Model file for the job. Use its own axes, mm. A direction names the side the tool comes from. Round coordinates to 2 decimals unless told otherwise and drop trailing zeros. Loops run counter-clockwise (first coordinate to the right, second up) from the corner with the lowest first, then second, coordinate; pieces in that order, holes last. Notation, with made-up numbers: M 24,-4 L 44,-4 A23 cw 44,14 Z; hole C 89.25,53 d11. An arc over 180 degrees is marked long. Use a Markdown table: item, result. Add a question column.
Q1. Pin check, flat tip, straight feed: pin 1 (1.5 mm diameter, centred on x = -14, z = 1.5, fed in from +Y). Stop position of the tip, or through.
Q2. Cut at C-C (z = 1.65). State how many separate pieces and enclosed holes the cut face has, plus the area to 3 significant figures.
Q3. Tool access for faces 1 (the face through (-8, 21, 3.175)), 2 (the face through (-30, 9.61, 2)): list every direction of +Z, -Z, +X, -X, +Y, -Y with a clear straight run to the whole face (end or side of a thin tool).
Q4. Cut at B-B (y = 31). Give the cut face in (x, z) (3 decimals), plus the area to 4 significant figures.
Q5. Mould opens along Y. For faces 3 (the face through (2, 28.698, 2)), 4 (the face through (-33, -8.54, 2)), 5 (the face through (-22.564, 38, 2)) say: +Y half, -Y half, draft (parallel to the pull), parting line (faces both ways), or undercut.
Q6. Cut at A-A (x = -21). Give the cut face in (y, z) (3 decimals), plus the area to 3 significant figures.
Q7. Probe line 1 (Y direction, x = -20.5, z = 2.15); line 2 (Y direction, x = -28.5, z = 2.75); line 3 (X direction, y = 16, z = 1.45). List the from-to ranges inside material, lowest first. Write a range as from..to.
from build123d import *

# Parameters (mm, degrees)
F0_W     = 8
F0_H     = 3.175
F0_R     = 1
F0_R_2   = 1.5
F0_W_2   = 3.175
F0_H_2   = 4
F0_W_3   = 12.5
F0_H_3   = 24
F0_W_4   = 6
F1_DEPTH = 3.175


# Not quite as in the source:
# - a length typed as a fraction of an inch, garbled in the dataset ("3 / 203.2 mm" for 3/8 in), is restored


with BuildPart() as f1:
    # F0 (on Top) → F1 (new body)
    with BuildSketch(Plane.XY):
        Polygon((-41.0637862384, -14.8897265702), (-7.5637862384, -14.8897265702), (25.9362137616, -14.8897265702), (25.9362137616, 28.6977734298), (-22.5637862384, 28.6977734298), (-22.5637862384, 46.6102734298), (-41.0637862384, 46.6102734298), align=None)
        with Locations((-33.0637862384, -10.1272265702)):
            Rectangle(F0_W, F0_H, mode=Mode.SUBTRACT)
        with Locations((-19.0637862384, -10.1272265702)):
            Rectangle(F0_W, F0_H, mode=Mode.SUBTRACT)
        with Locations((-31.8137862384, 13.6102734298)):
            Circle(F0_R, mode=Mode.SUBTRACT)
        Polygon((15.7612137616, -5.5397265702), (-38.0637862384, -5.5397265702), (-38.0637862384, 9.6102734298), (-22.5637862384, 9.6102734298), (-22.5637862384, 19.5227734298), (15.7612137616, 19.5227734298), (15.7612137616, 9.6102734298), align=None, mode=Mode.SUBTRACT)
        with BuildLine():
            ThreePointArc((-7.5637862384, -11.6272265702), (-8.6244464102, -9.0665663985), (-6.0637862384, -10.1272265702))
            ThreePointArc((-6.0637862384, -10.1272265702), (-6.5031260667, -11.187886742), (-7.5637862384, -11.6272265702))
        make_face(mode=Mode.SUBTRACT)
        with Locations((3.9362137616, -10.1272265702)):
            Rectangle(F0_W, F0_H, mode=Mode.SUBTRACT)
        with Locations((17.9362137616, -10.1272265702)):
            Rectangle(F0_W, F0_H, mode=Mode.SUBTRACT)
        with Locations((20.3487137616, -0.0397265702)):
            Circle(F0_R_2, mode=Mode.SUBTRACT)
        with Locations((20.3487137616, 6.4602734298)):
            Rectangle(F0_W_2, F0_H_2, mode=Mode.SUBTRACT)
        with Locations((-31.8137862384, 28.1102734298)):
            Rectangle(F0_W_3, F0_H_3, mode=Mode.SUBTRACT)
        with Locations((-31.8137862384, 42.6102734298)):
            Circle(F0_R, mode=Mode.SUBTRACT)
        with Locations((2.9362137616, 24.1102734298)):
            Rectangle(F0_W_4, F0_H, mode=Mode.SUBTRACT)
        with Locations((11.4362137616, 24.1102734298)):
            Circle(F0_R_2, mode=Mode.SUBTRACT)
        with Locations((19.9362137616, 24.1102734298)):
            Rectangle(F0_W_4, F0_H, mode=Mode.SUBTRACT)
    extrude(amount=F1_DEPTH)


solid = f1.part
Checked values:
| question | item | result |
|---|---|---|
| 1 | pin 1 | stops at y = 28.7 |
| 2 | separate pieces | 1 |
| 2 | enclosed holes | 14 |
| 2 | area | 1,580 mm^2 |
| 3 | face 1 | +Z, +X, -X, +Y, -Y |
| 3 | face 2 | +Z, -Z |
| 4 | outline | M -41.064,0 L -38.064,0 L -38.064,3.175 L -41.064,3.175 Z; M -25.564,0 L -22.564,0 L -22.564,3.175 L -25.564,3.175 Z |
| 4 | area | 19.05 mm^2 |
| 5 | face 3 | +Y half |
| 5 | face 4 | undercut |
| 5 | face 5 | draft |
| 6 | outline | M -14.89,0 L -11.715,0 L -11.715,3.175 L -14.89,3.175 Z; M -8.54,0 L -5.54,0 L -5.54,3.175 L -8.54,3.175 Z; M 19.523,0 L 28.698,0 L 28.698,3.175 L 19.523,3.175 Z |
| 6 | area | 48.7 mm^2 |
| 7 | line 1 | y = -14.89..-11.71, -8.54..-5.54, 19.52..28.7 |
| 7 | line 2 | y = -14.89..-5.54, 9.61..16.11, 40.11..46.61 |
| 7 | line 3 | x = -41.06..-22.56, 15.76..25.94 |
